Work out the finished part from the listing and answer in its coordinate system (mm). Face numbers are marked on the shaded views. A direction names the side the tool comes from. Coordinates: 2 decimals unless noted, no trailing zeros. Write each loop counter-clockwise with the first axis right and the second up, starting at its lowest first coordinate (ties: lowest second). Pieces come first, ordered by that corner, then holes. Notation, with made-up numbers: (67, 87.5) - (117, 87.5) arc R27 ccw to (117, 108.5) - close; hole circle Ø9 at (-38, 0.5). An arc over 180 degrees is marked (long way). Use one line per item in the form item = value. Start each with the question number.
Item 1: A cutting plane is placed at B-B (z = 20). Write down the section's boundary in (x, y).
Item 2: A cutting plane is placed at A-A (z = 5). Write down the section's boundary in (x, y), then the cut area to 3 significant figures.
Item 3: Given pin 1 (3.5 mm diameter, centred on y = 17, z = 27, fed in from +X); pin 2 (10 mm diameter, centred on x = 37, y = 13.5, fed in from +Z), each flat-ended and moving along its own axis, determine where each tip first touches the part or whether it passes through.
Item 4: A cutting plane is placed at C-C (y = 10). Give the number of separate pieces and of enclosed holes in the cut face, then the cut area to 3 significant figures.
Item 5: Determine the mould class of the marked faces 1, 2 and 3 for opening direction X: released by +X, released by -X, zero draft, split by the parting line, or undercut.
Item 6: A cutting plane is placed at D-D (x = 23.5). Write down the section's boundary in (y, z), then the cut area to 3 significant figures.
Item 7: Consider probe 1 along Z at (x, y) = (1.55, 10); probe 2 along Y at (x, z) = (28, 0.75); probe 3 along X at (y, z) = (14.25, 3). Determine where each line is inside the solid, lowest interval first.
Item 8: For the marked faces 4 and 5, determine the directions among +Z, -Z, +X, -X, +Y, -Y from which every point of the face is accessible in a straight line to the end or side of a thin tool.
Autodesk Fusion 360 part; units mm, degrees
sketch "草图1" plane through (0, 0, 0) normal (0, 0, 1) x (1, 0, 0)
  line L0 (0, 0) -> (56, 0)
  line L1 (56, 0) -> (56, 20)
  line L2 (56, 20) -> (0, 20)
  line L3 (0, 20) -> (0, 0)
  dimension "d1" = 56
  dimension "d2" = 20
extrude "拉伸1" add sketch "草图1" along normal blind 2 makes body 1
sketch "草图2" plane through (0, 0, 2) normal (0, 0, 1) x (-1, 0, 0)
  line L0 (0, -20) -> (0, 0)
  line L1 (0, 0) -> (-56, 0)
  line L2 (-56, 0) -> (-56, -20)
  line L3 (-56, -20) -> (0, -20)
  line L4 (-10, -10) -> (-50.5346, -10)
  line L5 (-28, -17) -> (-28, -4)
  circle A0 centre (-28, -10) radius 3
  circle A1 centre (-28, -10) radius 7 construction
  line L6 (-28, -10) -> (-35.6485, -17.6485) construction
  circle A2 centre (-32.9497, -14.9497) radius 1.6
  circle A3 centre (-23.0503, -14.9497) radius 1.6
  circle A4 centre (-23.0503, -5.0503) radius 1.6
  circle A5 centre (-32.9497, -5.0503) radius 1.6
  circle A6 centre (-42.9497, -14.9497) radius 1.6
  circle A7 centre (-42.9497, -5.0503) radius 1.6
  circle A8 centre (-13.0503, -14.9497) radius 1.6
  circle A9 centre (-13.0503, -5.0503) radius 1.6
  dimension "d5" = 6
  dimension "d6" = 14
  dimension "d7" = 45
  dimension "d8" = 3.2
  dimension "d10" = 360
  dimension "d13" = -10
  dimension "d14" = 3
extrude "拉伸2" cut sketch "草图2" against normal blind 2 contours L4 L5 A0 | L4 L5 A0 | L4 L5 A0 | L4 L5 A0 | A2 | A3 | A4 | A5 | A6 | A7 | A8 | A9 bodies 1
sketch "草图3" plane through (0, 0, 2) normal (0, 0, 1) x (-1, 0, 0)
  circle A0 centre (-42.9497, -14.9497) radius 1.6
  circle A1 centre (-23.0503, -14.9497) radius 1.6
  circle A2 centre (-13.0503, -5.0503) radius 1.6
  circle A3 centre (-32.9497, -14.9497) radius 1.6
  circle A4 centre (-42.9497, -5.0503) radius 1.6
  circle A5 centre (-28, -10) radius 3
  circle A6 centre (-13.0503, -14.9497) radius 1.6
  circle A7 centre (-23.0503, -5.0503) radius 1.6
  circle A8 centre (-32.9497, -5.0503) radius 1.6
  line L0 (0, -20) -> (0, 0)
  line L1 (0, 0) -> (-56, 0)
  line L2 (-56, 0) -> (-56, -20)
  line L3 (-56, -20) -> (0, -20)
  line L4 (0, 0) -> (-2, 0)
  line L5 (-2, 0) -> (-2, -20)
  line L6 (-2, -20) -> (0, -20)
  line L7 (0, -20) -> (0, 0)
  line L8 (-56, 0) -> (-54, 0)
  line L9 (-54, 0) -> (-54, -20)
  line L10 (-54, -20) -> (-56, -20)
  line L11 (-56, -20) -> (-56, 0)
  dimension "d17" = 2
  dimension "d18" = 2
extrude "拉伸3" add sketch "草图3" along normal blind 35 contours L0 L1 L3 L4 L5 L6 L7 | L1 L2 L3 L8 L9 L10 L11 bodies 1
fillet "圆角1" radius 1 4 edges at (56, 10, 0) (54, 10, 2) (2, 10, 2) (0, 10, 0) on bodies 1
sketch "草图4" plane through (56, 0, 0) normal (1, 0, 0) x (0, 1, 0)
  line L0 (0, 1) -> (20, 1)
  line L1 (20, 1) -> (20, 37)
  line L2 (20, 37) -> (0, 37)
  line L3 (0, 37) -> (0, 1)
  circle A0 centre (10, 27) radius 7 construction
  line L4 (0, 27) -> (0, 37)
  line L5 (20, 37) -> (20, 27)
  arc A1 (20, 26.9983) -> (0, 27) centre (10, 27) ccw
  line L6 (10, 27) -> (19, 27) construction
  circle A2 centre (17, 27) radius 1.6
  circle A3 centre (10, 34) radius 1.6
  circle A4 centre (3, 27) radius 1.6
  circle A5 centre (10, 20) radius 1.6
  circle A6 centre (10, 27) radius 3
  dimension "d23" = 14
  dimension "d24" = 27
  dimension "d25" = 20
  dimension "d26" = 3.2
  dimension "d28" = 360
  dimension "d29" = 6
extrude "拉伸4" cut sketch "草图4" against normal blind 56 contours L2 L3 L4 A1 | L1 L2 L5 A1 | A2 | A3 | A4 | A5 | A6 bodies 1
copy_body "实体->零部件1" bodies 1 removing the originals makes body 2 in component "Component'"
component "Component'" placed x (1, 0, 0) y (0, 1, 0) z (0, 0, 1) at (0, 0, 0)
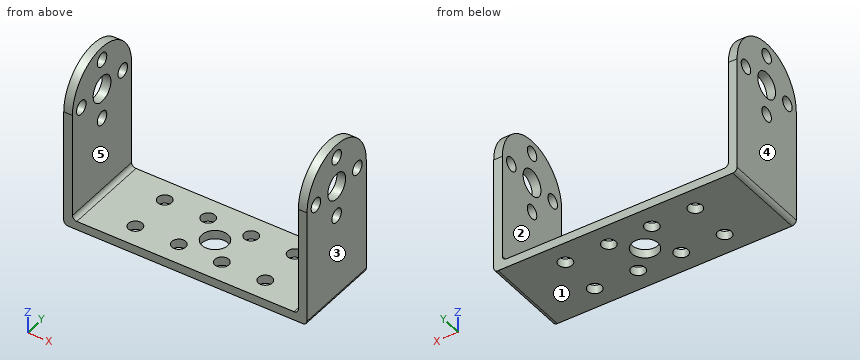
Answer:
q1.outline = (0, 0) - (2, 0) - (2, 8.4) - (0, 8.4) - close; (0, 11.6) - (2, 11.6) - (2, 20) - (0, 20) - close; (54, 0) - (56, 0) - (56, 8.4) - (54, 8.4) - close; (54, 11.6) - (56, 11.6) - (56, 20) - (54, 20) - close
q2.outline = (0, 0) - (2, 0) - (2, 20) - (0, 20) - close; (54, 0) - (56, 0) - (56, 20) - (54, 20) - close
q2.area = 80.0 mm²
q3.pin_1 = 56
q3.pin_2 = 2
q4.separate_pieces = 8
q4.enclosed_holes = 0
q4.area = 190 mm²
q5.face_1 = zero draft
q5.face_2 = undercut
q5.face_3 = released by +X
q6.outline = (0, 0) - (3.51, 0) - (3.51, 2) - (0, 2) - close; (6.59, 0) - (13.41, 0) - (13.41, 2) - (6.59, 2) - close; (16.49, 0) - (20, 0) - (20, 2) - (16.49, 2) - close
q6.area = 27.7 mm²
q7.probe_1 = 0 to 18.4, 21.6 to 24, 30 to 32.4, 35.6 to 37
q7.probe_2 = 0 to 7, 13 to 20
q7.probe_3 = 0 to 2, 54 to 56
q8.face_4 = +Z, -Z, -X, +Y, -Y
q8.face_5 = +Z, +Y, -Y
